The model under review builds one solid part; all positions refer to its coordinate system, in mm. Face numbers are marked on the shaded views. A direction names the side the tool comes from. Coordinates: 2 decimals unless noted, no trailing zeros. Write each loop counter-clockwise with the first axis right and the second up, starting at its lowest first coordinate (ties: lowest second). Pieces come first, ordered by that corner, then holes. Notation, with made-up numbers: M 24.5,-5.5 L 58.5,-5.5 A20 cw 58.5,23.5 Z; hole C 45,1.5 d8. An arc over 180 degrees is marked long. Answer as CSV lines item,"result". Start each with the question number.
from build123d import *

# Parameters (mm, degrees)
F0_R     = 1.5
F1_DEPTH = 60
F3_DEPTH = 36.401


with BuildPart() as f1:
    # F0 (on Top) → F1 (new body)
    with BuildSketch(Plane.XY):
        with BuildLine():
            Line((41.158495, -26.509628), (41.158495, 9.990372))
            Line((41.158495, 9.990372), (41.158495, 33.590372))
            Line((41.158495, 33.590372), (30.658495, 33.590372))
            Line((30.658495, 33.590372), (30.658495, 23.090372))
            Line((30.658495, 23.090372), (30.587656, 23.090927))
            ThreePointArc((30.587656, 23.090927), (22.898785, 15.521476), (15.329334, 23.210347))
            Line((15.329334, 23.210347), (15.258495, 23.210902))
            Line((15.258495, 23.210902), (15.258495, 33.590372))
            Line((15.258495, 33.590372), (4.758495, 33.590372))
            Line((4.758495, 33.590372), (4.758495, 9.990372))
            Line((4.758495, 9.990372), (4.758495, -26.509628))
            Line((4.758495, -26.509628), (41.158495, -26.509628))
        make_face()
        with Locations((7.697332, -23.348416)):
            Circle(F0_R, mode=Mode.SUBTRACT)
        with Locations((38.412604, -23.529183)):
            Circle(F0_R, mode=Mode.SUBTRACT)
        with Locations((7.79681, 7.112169)):
            Circle(F0_R, mode=Mode.SUBTRACT)
        with Locations((38.370336, 7.227415)):
            Circle(F0_R, mode=Mode.SUBTRACT)
    extrude(amount=F1_DEPTH)

    # F2 (on face) → F3 (cut, through all)
    with BuildSketch(Plane(origin=(4.758495, 0, 0), x_dir=(0, -1, 0), z_dir=(-1, 0, 0))):
        Polygon((26.509628, 60), (-28.34104, 60), (26.509628, 38.699873), align=None)
    extrude(amount=-F3_DEPTH, mode=Mode.SUBTRACT)


solid = f1.part
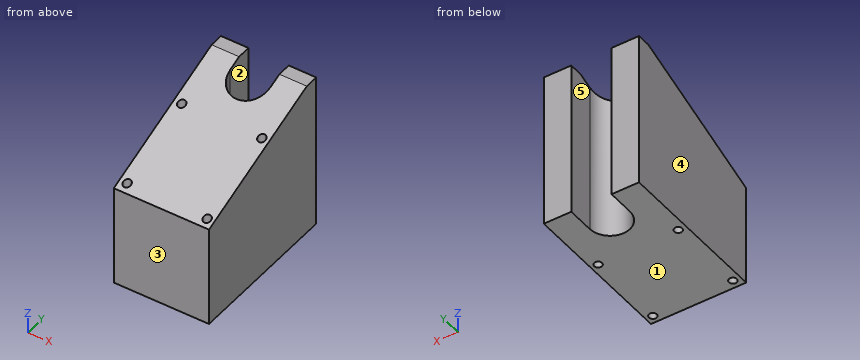
1) Clearance check with flat-ended pins moving along their axes: pin 1 Ø3.5 at (x, y) = (7.7, -23.35) entering from +Z; pin 2 Ø3.5 at (x, y) = (38.37, 7.23) entering from +Z; pin 3 Ø12 at (x, y) = (34.5, 0.5) entering from +Z. State where each tip first meets the part, or that it passes through.
2) Take a section at C-C on y = 22. Give the boundary of the cut face in (x, z).
3) Mouldability with a two-part tool opening along X and no side actions: class the marked faces 3, 4 and 5 as +X half, -X half, draft (parallel to the pull), parting line (faces both ways), or undercut.
4) Take a section at A-A on z = 49. Give the boundary of the cut face in (x, y), and give its area (3 significant figures).
5) Take a section at B-B on z = 26.5. Give the boundary of the cut face in (x, y), and give its area (3 significant figures).
6) To check wall thickness, follow line 1 (X direction, y = 30, z = 51); line 2 (X direction, y = 19.5, z = 37); line 3 (Y direction, x = 8.5, z = 7). State the ranges of each line that lie inside material, in increasing order. Write a range as [from, to].
7) Tool access review of the marked faces 1 and 2: name each direction out of +Z, -Z, +X, -X, +Y, -Y from which nothing blocks a thin tool from reaching the whole face with its end or side.
8) Take a section at D-D on x = 10.5. Give the boundary of the cut face in (y, z), and give its area (3 significant figures).
Results:
1,pin 1,"stops at z = 40.61"
1,pin 2,"stops at z = 52.48"
1,pin 3,"stops at z = 51.52"
2,outline,"M 4.76,0 L 15.42,0 L 15.42,57.54 L 4.76,57.54 Z; M 30.5,0 L 41.16,0 L 41.16,57.54 L 30.5,57.54 Z"
3,face 3,"draft"
3,face 4,"-X half"
3,face 5,"undercut"
4,outline,"M 4.76,0.01 L 41.16,0.01 L 41.16,33.59 L 30.66,33.59 L 30.66,23.09 L 30.59,23.09 A7.63 cw 15.33,23.21 L 15.26,23.21 L 15.26,33.59 L 4.76,33.59 Z; hole C 7.8,7.11 d3; hole C 38.37,7.23 d3"
4,area,"956 mm²"
5,outline,"M 4.76,-26.51 L 41.16,-26.51 L 41.16,33.59 L 30.66,33.59 L 30.66,23.09 L 30.59,23.09 A7.63 cw 15.33,23.21 L 15.26,23.21 L 15.26,33.59 L 4.76,33.59 Z; hole C 7.7,-23.35 d3; hole C 7.8,7.11 d3; hole C 38.37,7.23 d3; hole C 38.41,-23.53 d3"
5,area,"1,910 mm²"
6,line 1,"x = [4.76, 15.26], [30.66, 41.16]"
6,line 2,"x = [4.76, 16.26], [29.66, 41.16]"
6,line 3,"y = [-26.51, -24.62], [-22.08, 5.79], [8.44, 33.59]"
7,face 1,"-Z, +X, -X, +Y, -Y"
7,face 2,"+Z, -Z, +Y"
8,outline,"M -26.51,0 L 33.59,0 L 33.59,60 L 28.34,60 L -26.51,38.7 Z"
8,area,"3,020 mm²"
